from build123d import *

# Parameters (mm, degrees)
F0_R      = 7.95
F1_DEPTH  = 3.7
F2_R      = 8.75
F3_DEPTH  = 3.5
F4_R      = 7.95
F5_DEPTH  = 3.7
F6_R      = 1.157817429
F7_DEPTH  = 25
F8_R      = 1.150952134
F9_DEPTH  = 25
F10_R     = 7.150952134
F10_R_2   = 3
F10_R_3   = 1.05
F11_DEPTH = 7


with BuildPart() as f1:
    # F0 (on Top) → F1 (new body)
    with BuildSketch(Plane.XY):
        Circle(F0_R)
    extrude(amount=-F1_DEPTH)

    # F2 (on face) → F3 (join)
    with BuildSketch(Plane(origin=(0, 0, -3.7), x_dir=(1, 0, 0), z_dir=(0, 0, -1))):
        Circle(F2_R)
    extrude(amount=F3_DEPTH)

    # F4 (on face) → F5 (join)
    with BuildSketch(Plane(origin=(0, 0, -7.2), x_dir=(1, 0, 0), z_dir=(0, 0, -1))):
        Circle(F4_R)
    extrude(amount=F5_DEPTH)

    # F6 (on face) → F7 (cut)
    with BuildSketch(Plane(origin=(0, 0, -10.9), x_dir=(1, 0, 0), z_dir=(0, 0, -1))):
        with Locations((-5.9807905132, 0.4797341322)):
            Circle(F6_R)
        with Locations((2.5749333111, -5.4193835852)):
            Circle(F6_R)
        with Locations((3.4058572021, 4.939649453)):
            Circle(F6_R)
    extrude(amount=-F7_DEPTH, mode=Mode.SUBTRACT)

    # F8 (on face) → F9 (cut)
    with BuildSketch(Plane(origin=(0, 0, -10.9), x_dir=(1, 0, 0), z_dir=(0, 0, -1))):
        with Locations((-2.2553007404, 5.56000167)):
            Circle(F8_R)
        with Locations((5.9427530615, -0.8268531007)):
            Circle(F8_R)
        with Locations((-3.6874523211, -4.7331485693)):
            Circle(F8_R)
    extrude(amount=-F9_DEPTH, mode=Mode.SUBTRACT)

    # F10 (on face) → F11 (cut)
    with BuildSketch(Plane(origin=(0, 0, -10.9), x_dir=(1, 0, 0), z_dir=(0, 0, -1))):
        Circle(F10_R)
        Circle(F10_R_2, mode=Mode.SUBTRACT)
        Circle(F10_R_3)
    extrude(amount=-F11_DEPTH, mode=Mode.SUBTRACT)


solid = f1.part
Design review of the part built by this model. Coordinates are the model's own, in mm. A direction names the side the tool comes from. Round coordinates to 2 decimals unless told otherwise and drop trailing zeros. Write each loop counter-clockwise with the first axis right and the second up, starting at its lowest first coordinate (ties: lowest second). Pieces come first, ordered by that corner, then holes. Notation, with made-up numbers: (-32.5, -13) - (-4.5, -13) arc R23 cw to (-4.5, 3) - close; hole circle Ø1 at (-27.5, 82.5). An arc over 180 degrees is marked (long way). Use a Markdown table: item, result. Add a question column.
1. We need section A-A (y = 0). Count the separate pieces of the cut face and the enclosed holes in it, then the cut area to 3 significant figures.
2. Wall thickness on probe 1 along X at (y, z) = (0, -8.25); probe 2 along Y at (x, z) = (1.25, -4.5); probe 3 along Z at (x, y) = (3.5, 3.5): over which ranges is each line inside the solid? List them lowest first.
3. We need section D-D (x = 0). State the section outline as (y, z) points.
4. We need section B-B (x = 5.75). State the section outline as (y, z) points, then the cut area to 3 significant figures.
5. For faces 1 (the face through (-3.3, -0.1, -3.9)), 2 (the face through (-2.59, 4.39, -1.98)), 3 (the face through (2, 8, -3.7)), list the 3-axis set-ups (+Z, -Z, +X, -X, +Y, -Y) from which the entire face can be reached by the end or side of a thin tool; tool diameter is ignored.
6. Clearance check with flat-ended pins moving along their axes: pin 1 (5 mm diameter, centred on y = 3, z = -3, fed in from +X); pin 2 (1 mm diameter, centred on y = 1.5, z = -9.5, fed in from +X); pin 3 (3 mm diameter, centred on y = 4.5, z = -7.5, fed in from -X). State where each tip first meets the part, or that it passes through.
7. We need section C-C (z = -6.75). State the section outline as (x, y) points, then the cut area to 3 significant figures.
Output:
| question | item | result |
|---|---|---|
| 1 | separate pieces | 3 |
| 1 | enclosed holes | 0 |
| 1 | area | 91.6 mm2 |
| 2 | probe 1 | x = -7.95 to -7.15, -3 to -1.05, 1.05 to 3, 7.15 to 7.95 |
| 2 | probe 2 | y = -8.66 to -7.04, -2.73 to 2.73, 7.04 to 8.66 |
| 2 | probe 3 | z = -3.9 to 0 |
| 3 | outline | (-8.75, -7.2) - (-7.95, -7.2) - (-7.95, -10.9) - (-7.15, -10.9) - (-7.15, -3.9) - (-3, -3.9) - (-3, -10.9) - (-1.05, -10.9) - (-1.05, -3.9) - (1.05, -3.9) - (1.05, -10.9) - (3, -10.9) - (3, -3.9) - (7.15, -3.9) - (7.15, -10.9) - (7.95, -10.9) - (7.95, -7.2) - (8.75, -7.2) - (8.75, -3.7) - (7.95, -3.7) - (7.95, 0) - (-7.95, 0) - (-7.95, -3.7) - (-8.75, -3.7) - close |
| 4 | outline | (-6.6, -7.2) - (-5.49, -7.2) - (-5.49, -10.9) - (-4.25, -10.9) - (-4.25, -3.9) - (-0.31, -3.9) - (-0.31, 0) - (-5.49, 0) - (-5.49, -3.7) - (-6.6, -3.7) - close; (1.96, -3.9) - (4.25, -3.9) - (4.25, -10.9) - (5.49, -10.9) - (5.49, -7.2) - (6.6, -7.2) - (6.6, -3.7) - (5.49, -3.7) - (5.49, 0) - (1.96, 0) - close |
| 4 | area | 59.1 mm2 |
| 5 | face 1 | -Z |
| 5 | face 2 | +Z, -Z |
| 5 | face 3 | +Z |
| 6 | pin 1 | stops at x = 8.73 |
| 6 | pin 2 | stops at x = 7.89 |
| 6 | pin 3 | stops at x = -8.21 |
| 7 | outline | circle Ø17.5 at (0, 0); circle Ø6 at (0, 0); hole (-7.14, -0.43) arc R1.16 ccw to (-7.12, -0.71) arc R7.15 ccw to (3.95, -5.96) arc R1.16 ccw to (4.17, -5.81) arc R7.15 ccw to (3.19, 6.4) arc R1.16 ccw to (2.94, 6.52) arc R7.15 ccw to start; hole circle Ø2.1 at (0, 0) |
| 7 | area | 105 mm2 |
